The listing builds one solid part. Answer for the finished solid, in the listing's coordinates (mm). Round coordinates to 2 decimals unless told otherwise and drop trailing zeros. Order: outer loops, then holes, each group sorted by start corner. A loop starts at its lowest first (then second) coordinate and runs counter-clockwise, first axis right, second up. Notation, with made-up numbers: (57, 78.25) -> (103, 78.25) arc R9 cw to (103, 82.25) -> close; hole circle Ø7 at (9, -33). An arc over 180 degrees is marked (long way). Return JSON: item names as keys, results as strings. Group by question number.
(1) The part is cut by section B-B (z = 0). Determine the outline of the cut face in (x, y).
(2) Consider line 1 (X direction, y = 4, z = 0); line 2 (X direction, y = 9.25, z = 2.25); line 3 (Z direction, x = -4.75, y = 7.5). Determine where each line is inside the solid, lowest interval first. Write a range as [from, to].
(3) The part is cut by section C-C (y = 2.5). Determine the outline of the cut face in (x, z).
(4) The part is cut by section A-A (x = 0). Determine the outline of the cut face in (y, z).
(5) Determine the mould class of faces 1 (the face through (2, 10.23, 2)), 2 (the face through (-2.44, 5.04, -0.54)), 3 (the face through (11.848, 5.071, -1.556)) for opening direction Z: +Z half, -Z half, draft (parallel to the pull), parting line (faces both ways), or undercut.
(6) Each of these flat-tipped pins is pushed along its axis until it touches: pin 1 (5 mm diameter, centred on x = 5.5, z = 3.5, fed in from -Y); pin 2 (3 mm diameter, centred on x = 0, z = 0, fed in from +Y); pin 3 (1 mm diameter, centred on x = -7, y = 5, fed in from -Z); pin 4 (1.5 mm diameter, centred on y = 8, z = 2, fed in from -X). Where does it stop, or does it pass through?
from build123d import *

# Parameters (mm, degrees)
SKETCH1_R           = 11.95
SKETCH1_R_2         = 7.985
BOSS_EXTRUDE1_DEPTH = 10.23
CHAMFER1_SIZE       = 2
SKETCH2_R           = 7.985
SKETCH2_R_2         = 2.5
BOSS_EXTRUDE3_DEPTH = 10.23


with BuildPart() as part:
    # Sketch1 → Boss-Extrude1 (new body)
    with BuildSketch(Plane(origin=(0, 0, 0), x_dir=(1, 0, 0), z_dir=(0, 1, 0))):
        with Locations(Location((0, 0, 0), (0, 0, 270))):
            Circle(SKETCH1_R)
        with Locations(Location((0, 0, 0), (0, 0, 270))):
            Circle(SKETCH1_R_2, mode=Mode.SUBTRACT)
    extrude(amount=BOSS_EXTRUDE1_DEPTH)

    # Chamfer1
    chamfer1_edges = [part.edges().sort_by_distance(p)[0] for p in [
        (0, 0, -11.95),
        (0, 10.23, -11.95),
    ]]
    chamfer(chamfer1_edges, length=CHAMFER1_SIZE)

    # Sketch2 → Boss-Extrude3 (add)
    with BuildSketch(Plane(origin=(0, 0, 0), x_dir=(1, 0, 0), z_dir=(0, 1, 0))):
        Circle(SKETCH2_R)
        with Locations(Location((0, 0, 0), (0, 0, 270))):
            Circle(SKETCH2_R_2, mode=Mode.SUBTRACT)
    extrude(amount=BOSS_EXTRUDE3_DEPTH)


solid = part.part
Answer below:
{
 "1": {"outline": "(-11.95, 2) -> (-9.95, 0) -> (-2.5, 0) -> (-2.5, 10.23) -> (-9.95, 10.23) -> (-11.95, 8.23) -> close; (2.5, 0) -> (9.95, 0) -> (11.95, 2) -> (11.95, 8.23) -> (9.95, 10.23) -> (2.5, 10.23) -> close"},
 "2": {"line 1": "x = [-11.95, -2.5], [2.5, 11.95]", "line 2": "x = [-10.7, -1.09], [1.09, 10.7]", "line 3": "z = [-10.97, 10.97]"},
 "3": {"outline": "circle Ø23.9 at (0, 0); hole circle Ø5 at (0, 0)"},
 "4": {"outline": "(0, -9.95) -> (2, -11.95) -> (8.23, -11.95) -> (10.23, -9.95) -> (10.23, -2.5) -> (0, -2.5) -> close; (0, 2.5) -> (10.23, 2.5) -> (10.23, 9.95) -> (8.23, 11.95) -> (2, 11.95) -> (0, 9.95) -> close"},
 "5": {"face 1": "draft", "face 2": "undercut", "face 3": "parting line"},
 "6": {"pin 1": "stops at y = 0", "pin 2": "passes through", "pin 3": "stops at z = -10.03", "pin 4": "stops at x = -11.88"}
}
